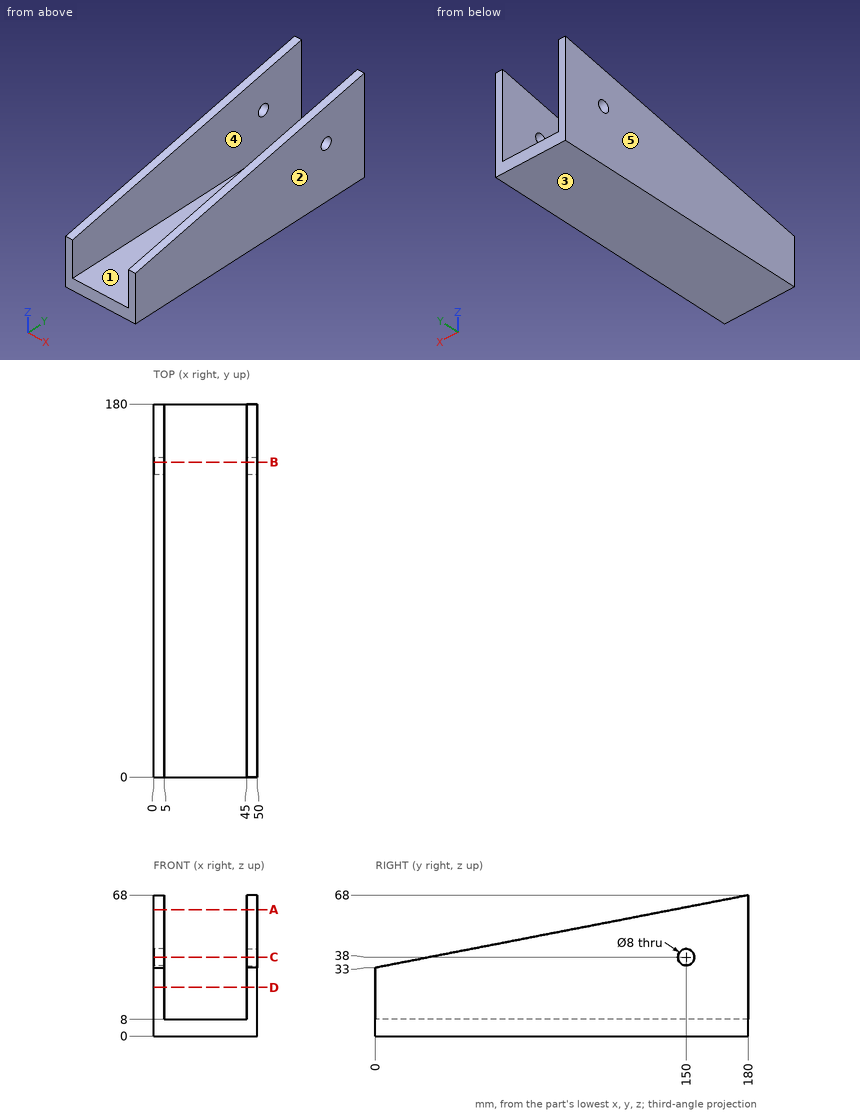
Can you work these out from the drawing? Everything is in mm from the part's minimum corner. A direction names the side the tool comes from. Give positions to 0.01 mm unless a question says otherwise; leave off trailing zeros. Write each loop counter-clockwise with the first axis right and the second up, starting at its lowest first coordinate (ties: lowest second). Pieces come first, ordered by that corner, then holes. Notation, with made-up numbers: (2, 23) -> (7, 23) arc R30 ccw to (7, 59) -> close; hole circle Ø4 at (-4.5, 69). An arc over 180 degrees is marked (long way). Write each question's results on one line, items separated by ' | '.
Item 1: For pin 1 Ø6 at (x, z) = (37, 7) entering from -Y; pin 2 Ø10 at (x, y) = (8.5, 131.5) entering from +Z; pin 3 Ø8 at (x, y) = (31, 156.5) entering from +Z; pin 4 Ø1.5 at (x, z) = (44, 48) entering from +Y, each with a flat end and sliding along its axis, tell me the tip position at first contact or that it passes through.
Output:
pin 1: stops at y = 0 | pin 2: stops at z = 59.26 | pin 3: stops at z = 8 | pin 4: passes through
Item 2: On a 3-axis mill with a long thin cutter (end or side, diameter ignored), from which of +Z, -Z, +X, -X, +Y, -Y can I reach the whole of each face in a straight line? I mean the marked faces 1 and 2. Say none if no direction works.
Output:
face 1: +Z, +Y, -Y | face 2: +Z, -Z, +X, +Y, -Y
Item 3: Suppose I cut it at C-C on z = 38. Write out the boundary of the cut face in (x, y).
Output:
outline: (0, 25.71) -> (5, 25.71) -> (5, 146) -> (0, 146) -> close; (0, 154) -> (5, 154) -> (5, 180) -> (0, 180) -> close; (45, 25.71) -> (50, 25.71) -> (50, 146) -> (45, 146) -> close; (45, 154) -> (50, 154) -> (50, 180) -> (45, 180) -> close
Item 4: We'd pull the mould along X, two halves only. Please class the marked faces 3, 4 and 5: pulls with the +X half, pulls with the -X half, needs draft (parallel to the pull), parting line crosses it, or undercut.
Output:
face 3: needs draft | face 4: undercut | face 5: pulls with the -X half
Item 5: Suppose I cut it at A-A on z = 61. Write out the boundary of the cut face in (x, y), plus the area to 3 significant figures.
Output:
outline: (0, 144) -> (5, 144) -> (5, 180) -> (0, 180) -> close; (45, 144) -> (50, 144) -> (50, 180) -> (45, 180) -> close | area: 360 mm^2
Item 6: If I drill on L1, parallel to X at y = 71, z = 22; L2, parallel to Z at x = 2, y = 150; L3, parallel to Z at x = 38, y = 117, over which ranges is the centre line in solid material (lowest first)?
Output:
L1: x = 0 to 5, 45 to 50 | L2: z = 0 to 34, 42 to 62.17 | L3: z = 0 to 8
Item 7: Suppose I cut it at D-D on z = 23.5. Write out the boundary of the cut face in (x, y).
Output:
outline: (0, 0) -> (5, 0) -> (5, 180) -> (0, 180) -> close; (45, 0) -> (50, 0) -> (50, 180) -> (45, 180) -> close
Item 8: Suppose I cut it at B-B on y = 152. Write out the boundary of the cut face in (x, z).
Output:
outline: (0, 0) -> (50, 0) -> (50, 34.54) -> (45, 34.54) -> (45, 8) -> (5, 8) -> (5, 34.54) -> (0, 34.54) -> close; (0, 41.46) -> (5, 41.46) -> (5, 62.56) -> (0, 62.56) -> close; (45, 41.46) -> (50, 41.46) -> (50, 62.56) -> (45, 62.56) -> close
